Source: CAD feature listing. Evaluate the final solid. Frame: model axes, mm. Round coordinates to 2 decimals unless told otherwise and drop trailing zeros. Order: outer loops, then holes, each group sorted by start corner. A loop starts at its lowest first (then second) coordinate and runs counter-clockwise, first axis right, second up.
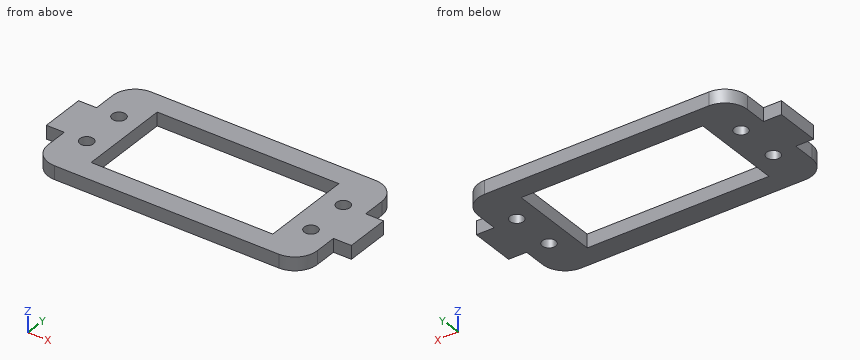
```python
from build123d import *

# Parameters (mm, degrees)
SALIENTE_EXTRUIR1_DEPTH = 3
CORTAR_EXTRUIR1_REACH   = 5
CROQUIS2_R              = 1.505219631
CROQUIS2_W              = 40.5
CROQUIS2_H              = 20.5
REDONDEO1_R             = 5


with BuildPart() as part:
    # Croquis1 → Saliente-Extruir1 (new body)
    with BuildSketch(Plane.XY):
        Polygon((-30, -5), (-30, -15), (30, -15), (30, -5), (34, -5), (34, 5), (30, 5), (30, 15), (-30, 15), (-30, 5), (-34, 5), (-34, -5), align=None)
    extrude(amount=SALIENTE_EXTRUIR1_DEPTH)

    # Croquis2 → Cortar-Extruir1 (cut, up to next)
    with BuildSketch(Plane.XY.offset(3), mode=Mode.PRIVATE) as cortar_extruir1_sk1:
        with Locations((25, 5)):
            Circle(CROQUIS2_R)
    cortar_extruir1_tool1 = extrude(cortar_extruir1_sk1.sketch, amount=-CORTAR_EXTRUIR1_REACH, mode=Mode.PRIVATE) & part.part
    add(cortar_extruir1_tool1.solids().sort_by_distance((25, 5, 3))[0], mode=Mode.SUBTRACT)
    # Croquis2 → Cortar-Extruir1 (cut, up to next)
    with BuildSketch(Plane.XY.offset(3), mode=Mode.PRIVATE) as cortar_extruir1_sk2:
        with Locations((-25, 5)):
            Circle(CROQUIS2_R)
    cortar_extruir1_tool2 = extrude(cortar_extruir1_sk2.sketch, amount=-CORTAR_EXTRUIR1_REACH, mode=Mode.PRIVATE) & part.part
    add(cortar_extruir1_tool2.solids().sort_by_distance((-25, 5, 3))[0], mode=Mode.SUBTRACT)
    # Croquis2 → Cortar-Extruir1 (cut, up to next)
    with BuildSketch(Plane.XY.offset(3), mode=Mode.PRIVATE) as cortar_extruir1_sk3:
        with Locations((25, -5)):
            Circle(CROQUIS2_R)
    cortar_extruir1_tool3 = extrude(cortar_extruir1_sk3.sketch, amount=-CORTAR_EXTRUIR1_REACH, mode=Mode.PRIVATE) & part.part
    add(cortar_extruir1_tool3.solids().sort_by_distance((25, -5, 3))[0], mode=Mode.SUBTRACT)
    # Croquis2 → Cortar-Extruir1 (cut, up to next)
    with BuildSketch(Plane.XY.offset(3), mode=Mode.PRIVATE) as cortar_extruir1_sk4:
        with Locations((-25, -5)):
            Circle(CROQUIS2_R)
    cortar_extruir1_tool4 = extrude(cortar_extruir1_sk4.sketch, amount=-CORTAR_EXTRUIR1_REACH, mode=Mode.PRIVATE) & part.part
    add(cortar_extruir1_tool4.solids().sort_by_distance((-25, -5, 3))[0], mode=Mode.SUBTRACT)
    # Croquis2 → Cortar-Extruir1 (cut, up to next)
    with BuildSketch(Plane.XY.offset(3), mode=Mode.PRIVATE) as cortar_extruir1_sk5:
        Rectangle(CROQUIS2_W, CROQUIS2_H)
    cortar_extruir1_tool5 = extrude(cortar_extruir1_sk5.sketch, amount=-CORTAR_EXTRUIR1_REACH, mode=Mode.PRIVATE) & part.part
    add(cortar_extruir1_tool5.solids().sort_by_distance((0, 0, 3))[0], mode=Mode.SUBTRACT)

    # Redondeo1
    redondeo1_edges = [part.edges().sort_by_distance(p)[0] for p in [
        (30, -15, 1.5),
        (-30, -15, 1.5),
        (-30, 15, 1.5),
        (30, 15, 1.5),
    ]]
    fillet(redondeo1_edges, radius=REDONDEO1_R)


solid = part.part
```
1. Section C-C on x = 17.5. Return loops of the section in (y, z), plus the area to 3 significant figures.
2. Section A-A on y = 2.75. Return loops of the section in (x, z), plus the area to 3 significant figures.
3. Line query: line 1 along Y through (x, z) = (25, 1.65); line 2 along Y through (x, z) = (15, 0.65); line 3 along X through (y, z) = (9.25, 2.45). Output: solid intervals per line, ascending.
4. Section B-B on z = 0.75. Return loops of the section in (x, y), plus the area to 4 significant figures.
5. First-contact query: pin 1 (0.9 mm diameter, centred on y = -8, z = 1.5, fed in from +X); pin 2 (1.5 mm diameter, centred on x = 31, z = 1, fed in from -Y); pin 3 (1.5 mm diameter, centred on x = -31.5, z = 1, fed in from +Y). Flat tips, straight axial feed; report the tip coordinate or a pass-through.
Result:
1. outline: (-15, 0) - (-10.25, 0) - (-10.25, 3) - (-15, 3) - close; (10.25, 0) - (15, 0) - (15, 3) - (10.25, 3) - close
1. area: 28.5 mm2
2. outline: (-34, 0) - (-20.25, 0) - (-20.25, 3) - (-34, 3) - close; (20.25, 0) - (34, 0) - (34, 3) - (20.25, 3) - close
2. area: 82.5 mm2
3. line 1: y = -15 to -6.51, -3.49 to 3.49, 6.51 to 15
3. line 2: y = -15 to -10.25, 10.25 to 15
3. line 3: x = -30 to -20.25, 20.25 to 30
4. outline: (-34, -5) - (-30, -5) - (-30, -10) arc R5 ccw to (-25, -15) - (25, -15) arc R5 ccw to (30, -10) - (30, -5) - (34, -5) - (34, 5) - (30, 5) - (30, 10) arc R5 ccw to (25, 15) - (-25, 15) arc R5 ccw to (-30, 10) - (-30, 5) - (-34, 5) - close; hole circle Ø3.01 at (-25, -5); hole circle Ø3.01 at (-25, 5); hole (-20.25, -10.25) - (20.25, -10.25) - (20.25, 10.25) - (-20.25, 10.25) - close; hole circle Ø3.01 at (25, -5); hole circle Ø3.01 at (25, 5)
4. area: 1,000 mm2
5. pin 1: stops at x = 30
5. pin 2: stops at y = -5
5. pin 3: stops at y = 5
